```python
from build123d import *

# Parameters (mm, degrees)
BOSS_EXTRU_1_DEPTH           = 15
ESQUISSE3_R                  = 5
ENL_V_MAT_EXTRU_1_DEPTH      = 390.991583511
R_P_TITION_CIRCULAIRE1_COUNT = 4


with BuildPart() as part:
    # Esquisse1 → Boss.-Extru.1 (new body)
    with BuildSketch(Plane.XY):
        with BuildLine():
            Line((-309.678238443, -150), (190.321761557, -150))
            ThreePointArc((190.321761557, -150), (225.677100616, -135.355339059), (240.321761557, -100))
            Line((240.321761557, -100), (240.321761557, 100))
            ThreePointArc((240.321761557, 100), (225.677100616, 135.355339059), (190.321761557, 150))
            Line((190.321761557, 150), (-309.678238443, 150))
            ThreePointArc((-309.678238443, 150), (-345.033577502, 135.355339059), (-359.678238443, 100))
            Line((-359.678238443, 100), (-359.678238443, -100))
            ThreePointArc((-359.678238443, -100), (-345.033577502, -135.355339059), (-309.678238443, -150))
        make_face()
    extrude(amount=BOSS_EXTRU_1_DEPTH)

    # Esquisse3 → Enl_v. mat.-Extru.1 (cut, through all)
    with BuildSketch(Plane.XY.offset(15)):
        with Locations((-293.418714055, 83.447366527)):
            Circle(ESQUISSE3_R)
        Polygon((-263.366675854, 124.106006445), (-252.760074137, 113.499404727), (-266.90220976, 99.357269104), (-277.508811478, 109.963870821), align=None)
        Polygon((-309.328616632, 56.930862233), (-319.935218349, 67.53746395), (-334.077353973, 53.395328327), (-323.470752255, 42.788726609), align=None)
    enl_v_mat_extru_1 = extrude(amount=-ENL_V_MAT_EXTRU_1_DEPTH, mode=Mode.SUBTRACT)

    # R_p_tition circulaire1: Enl_v. mat.-Extru.1 ×4 about axis
    r_p_tition_circulaire1_axis = Axis((-209.678238443, 0, 0), (0, 0, 1))
    for i in range(1, R_P_TITION_CIRCULAIRE1_COUNT):
        add(enl_v_mat_extru_1.rotate(r_p_tition_circulaire1_axis, i * 360 / R_P_TITION_CIRCULAIRE1_COUNT), mode=Mode.SUBTRACT)


solid = part.part
```
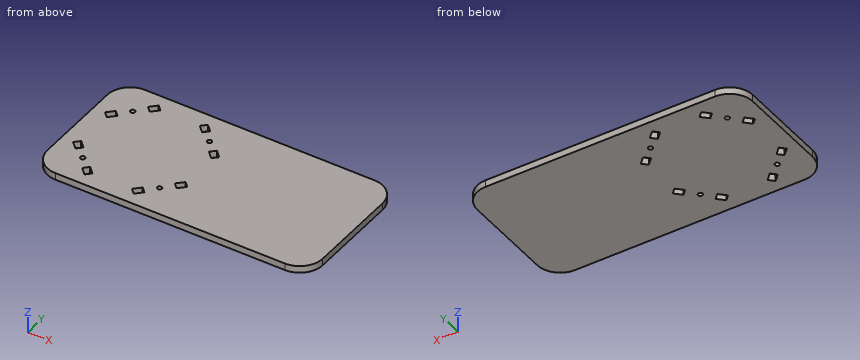
Check sheet for the modelled part. Datum: model origin and axes. Units: mm. Coordinates: 2 decimals unless noted, no trailing zeros.
1) Gauge pin test, flat ends, axial feed: pin 1 (1 mm diameter, centred on y = 101, z = 9, fed in from +X); pin 2 (6 mm diameter, centred on x = -293.42, y = 83.45, fed in from -Z). Record the tip position at first contact, or that the pin passes through.
2) Material ranges on probe 1 along Y at (x, z) = (-274, 3); probe 2 along Y at (x, z) = (-318, 9); probe 3 along X at (y, z) = (47.5, 13), recorded low to high.
3) Sectioned sample at A-A (z = 3.5). Count the separate pieces of the cut face and the enclosed holes in it, and give its area (3 significant figures).
Check sheet entries:
1. pin 1: stops at x = 240.32
1. pin 2: passes through
2. probe 1: y = -150 to -113.47, -107.04 to 106.46, 113.47 to 150
2. probe 2: y = -149.3 to -66.19, -48.26 to 48.26, 65.6 to 149.3
2. probe 3: x = -359.68 to -328.18, -318.76 to -100.6, -91.76 to 240.32
3. separate pieces: 1
3. enclosed holes: 12
3. area: 175,000 mm2
